The figure shows three views and two pictorial views of one solid part (mm, origin at its lowest corner). Answer the questions. A direction names the side the tool comes from. Give positions to 0.01 mm unless a question says otherwise; leave off trailing zeros. Order: outer loops, then holes, each group sorted by start corner. A loop starts at its lowest first (then second) coordinate and runs counter-clockwise, first axis right, second up. Notation, with made-up numbers: (5, 35) -> (52, 35) arc R26 cw to (52, 58) -> close; hole circle Ø5 at (78.25, 17.5). An arc over 180 degrees is marked (long way). Use one line per item in the form item = value.
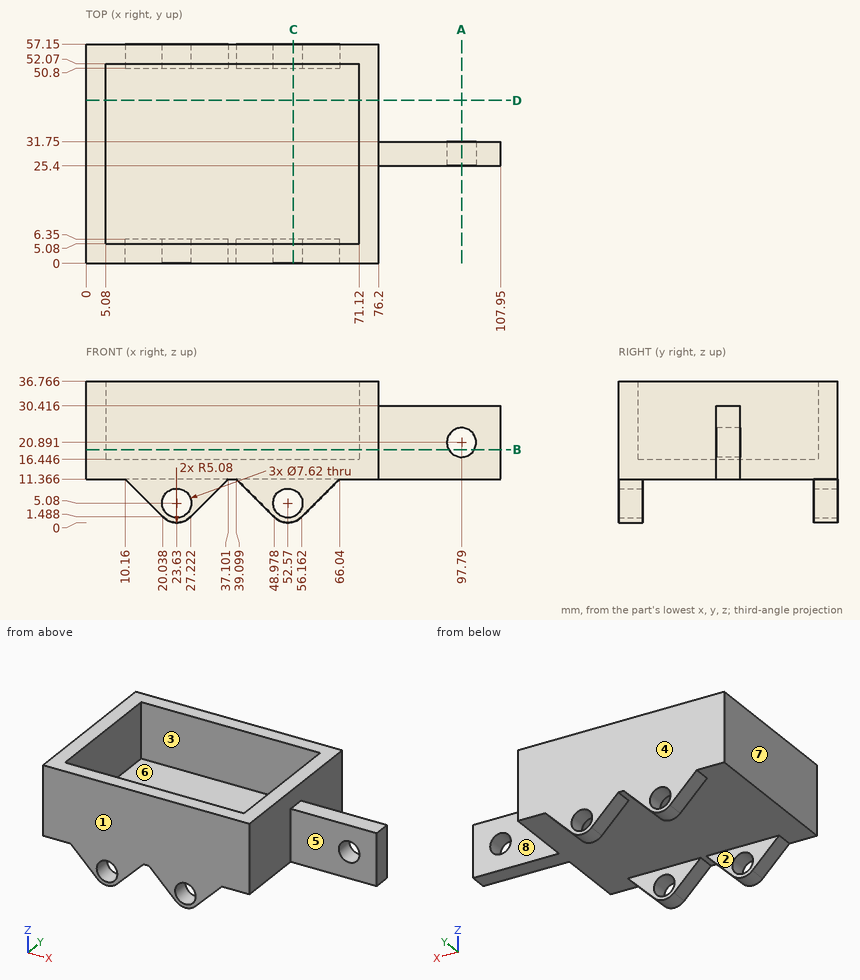
Item 1: Determine the mould class of the marked faces 6, 7 and 8 for opening direction X: +X half, -X half, draft (parallel to the pull), parting line (faces both ways), or undercut.
Checks:
face_6 = undercut
face_7 = -X half
face_8 = draft
Item 2: Which of the six approach directions +Z, -Z, +X, -X, +Y, -Y give full straight-line access (tool end or side, diameter ignored) to the marked faces 1, 2, 3, 4 and 5?
Checks:
face_1 = +Z, -Z, +X, -X, -Y
face_2 = -Z, +X, -X
face_3 = +Z
face_4 = +Z, -Z, +X, -X, +Y
face_5 = +Z, -Z, +X, -Y
Item 3: Straight lines are drawn through the part: L1, parallel to X at y = 35, z = 33; L2, parallel to Z at x = 97.79, y = 27.25; L3, parallel to Y at x = 21, z = 16.5. For each, find the intervals that lie inside material, in ascending order. Write a range as from..to.
Checks:
L1 = 0..5.08, 71.12..76.2
L2 = 11.37..17.08, 24.7..30.42
L3 = 0..5.08, 52.07..57.15
Item 4: Given pin 1 Ø12 at (x, y) = (12.5, 43) entering from -Z; pin 2 Ø10 at (x, z) = (37.5, 5) entering from +Y; pin 3 Ø4.5 at (x, z) = (52.57, 5.08) entering from -Y; pin 4 Ø10 at (y, z) = (7, 11.5) entering from +X, each flat-ended and moving along its own axis, determine where each tip first touches the part or whether it passes through.
Checks:
pin_1 = 11.37
pin_2 = 57.15
pin_3 = through
pin_4 = 76.2
Item 5: The part is cut by section C-C on x = 54. State how many separate pieces and enclosed holes the cut face has, and give its area (3 significant figures).
Checks:
separate_pieces = 3
enclosed_holes = 0
area = 549 mm²
Item 6: The part is cut by section A-A on x = 97.79. Give the vertices of the cut face in (y, z).
Checks:
outline = (25.4, 11.37) -> (31.75, 11.37) -> (31.75, 17.08) -> (25.4, 17.08) -> close; (25.4, 24.7) -> (31.75, 24.7) -> (31.75, 30.42) -> (25.4, 30.42) -> close
Item 7: The part is cut by section D-D on y = 42.5. Give the vertices of the cut face in (x, z).
Checks:
outline = (0, 11.37) -> (76.2, 11.37) -> (76.2, 36.77) -> (71.12, 36.77) -> (71.12, 16.45) -> (5.08, 16.45) -> (5.08, 36.77) -> (0, 36.77) -> close
Item 8: The part is cut by section B-B on z = 19. Give the vertices of the cut face in (x, y).
Checks:
outline = (0, 0) -> (76.2, 0) -> (76.2, 25.4) -> (94.48, 25.4) -> (94.48, 31.75) -> (76.2, 31.75) -> (76.2, 57.15) -> (0, 57.15) -> close; (101.1, 25.4) -> (107.95, 25.4) -> (107.95, 31.75) -> (101.1, 31.75) -> close; hole (5.08, 5.08) -> (71.12, 5.08) -> (71.12, 52.07) -> (5.08, 52.07) -> close
